```python
from build123d import *

# Parameters (mm, degrees)
SKETCH1_W                 = 22
SKETCH1_H                 = 22
BOSS_EXTRUDE1_DEPTH       = 3.175
SKETCH2_R                 = 5
CUT_EXTRUDE1_DEPTH        = 16.877047112
CHAMFER1_SIZE             = 0.5
F_3_0MM_DOWEL_HOLE1_D     = 3.3
F_3_0MM_DOWEL_HOLE1_DEPTH = 5
F_3_0MM_DOWEL_HOLE1_TIP   = 0.991420021


with BuildPart() as part:
    # Sketch1 → Boss-Extrude1 (new body)
    with BuildSketch(Plane(origin=(0, 0, 0), x_dir=(1, 0, 0), z_dir=(0, 1, 0))):
        Rectangle(SKETCH1_W, SKETCH1_H)
    extrude(amount=BOSS_EXTRUDE1_DEPTH)

    # Sketch2 → Cut-Extrude1 (cut, through all)
    with BuildSketch(Plane(origin=(0, 3.175, 0), x_dir=(1, 0, 0), z_dir=(0, 1, 0))):
        with Locations(Location((0, 0, 0), (0, 0, 270))):
            Circle(SKETCH2_R)
    extrude(amount=-CUT_EXTRUDE1_DEPTH, mode=Mode.SUBTRACT)

    # Chamfer1
    chamfer1_edges = [part.edges().sort_by_distance(p)[0] for p in [
        (11, 1.5875, 11),
        (-11, 1.5875, 11),
        (-11, 1.5875, -11),
        (11, 1.5875, -11),
    ]]
    chamfer(chamfer1_edges, length=CHAMFER1_SIZE)

    # Ø3.0mm Dowel Hole1
    with Locations(Plane(origin=(0, 3.175, 0), x_dir=(1, 0, 0), z_dir=(0, 1, 0))):
        with Locations((0, 8), (8, 0), (0, -8), (-8, 0)):
            Hole(F_3_0MM_DOWEL_HOLE1_D / 2, depth=F_3_0MM_DOWEL_HOLE1_DEPTH)
            with Locations((0, 0, -(F_3_0MM_DOWEL_HOLE1_DEPTH + F_3_0MM_DOWEL_HOLE1_TIP / 2))):  # 118° drill point
                Cone(0, F_3_0MM_DOWEL_HOLE1_D / 2, F_3_0MM_DOWEL_HOLE1_TIP, mode=Mode.SUBTRACT)


solid = part.part
```
The model under review builds one solid part; all positions refer to its coordinate system, in mm. Coordinates: 2 decimals unless noted, no trailing zeros. Order: outer loops, then holes, each group sorted by start corner. A loop starts at its lowest first (then second) coordinate and runs counter-clockwise, first axis right, second up. Notation, with made-up numbers: M -27,53.5 L 20,53.5 A14 ccw 20,59.5 Z; hole C 22.25,57.25 d2. An arc over 180 degrees is marked long. One line per question, with ' | ' between items.
(1) Add section D-D, the plane z = 0. Write out the cut boundary in (x, y) (3 decimals).
Geometry results:
outline: M -11,0 L -9.65,0 L -9.65,3.175 L -11,3.175 Z; M -6.35,0 L -5,0 L -5,3.175 L -6.35,3.175 Z; M 5,0 L 6.35,0 L 6.35,3.175 L 5,3.175 Z; M 9.65,0 L 11,0 L 11,3.175 L 9.65,3.175 Z
(2) Add section C-C, the plane y = 1.15. Write out the cut boundary in (x, z), then the cut area to 3 significant figures.
Geometry results:
outline: M -11,-10.5 L -10.5,-11 L 10.5,-11 L 11,-10.5 L 11,10.5 L 10.5,11 L -10.5,11 L -11,10.5 Z; hole C -8,0 d3.3; hole C 0,0 d10; hole C 0,-8 d3.3; hole C 0,8 d3.3; hole C 8,0 d3.3 | area: 371 mm²
(3) Insertion check: pin 1 (3 mm diameter, centred on x = 0, z = 8, fed in from +Y). The pin has a flat end and moves straight along its axis. Give the tip position at first contact, or say it passes through.
Geometry results:
pin 1: passes through
(4) Add section A-A, the plane x = 3. Write out the cut boundary in (y, z) (3 decimals).
Geometry results:
outline: M 0,-11 L 3.175,-11 L 3.175,-4 L 0,-4 Z; M 0,4 L 3.175,4 L 3.175,11 L 0,11 Z
(5) The part is to be moulded in two halves that separate along Z. For faces 1 (the face through (1.31, 1.57, 9)), 2 (the face through (-5, 3.175, -3)), 3 (the face through (0, 2, -11)), 4 (the face through (-4.88, 1.61, -1.08)), say which applies: +Z half, -Z half, draft (parallel to the pull), parting line (faces both ways), or undercut.
Geometry results:
face 1: undercut | face 2: draft | face 3: -Z half | face 4: undercut
(6) For probe 1 along Z at (x, y) = (8, 1.7); probe 2 along X at (y, z) = (1.25, 3.25), list the stretches that pass through material, from the lowest coordinate up. Write a range as from..to.
Geometry results:
probe 1: z = -11..-1.65, 1.65..11 | probe 2: x = -11..-3.8, 3.8..11
(7) Add section B-B, the plane z = -8. Write out the cut boundary in (x, y) (3 decimals), then the cut area to 3 significant figures.
Geometry results:
outline: M -11,0 L -1.65,0 L -1.65,3.175 L -11,3.175 Z; M 1.65,0 L 11,0 L 11,3.175 L 1.65,3.175 Z | area: 59.4 mm²
